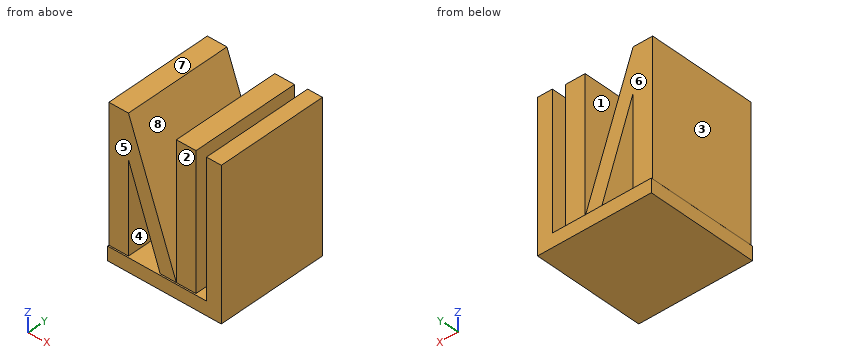
from build123d import *

# Parameters (mm, degrees)
F0_W     = 114.3
F0_H     = 152.4
F1_DEPTH = 15.24
F2_W     = 101.6
F2_H     = 14.1224
F3_DEPTH = 57.15
F4_DEPTH = 57.15
F5_W     = 20.146407
F5_H     = 137.283351
F6_DEPTH = 55.626
F7_DEPTH = 55.626


with BuildPart() as f1:
    # F0 (on Right) → F1 (new body)
    with BuildSketch(Plane.YZ):
        Rectangle(F0_W, F0_H)
    extrude(amount=F1_DEPTH)

    # F2 (on Front) → F3 (join)
    with BuildSketch(Plane.XZ):
        with Locations((-50.8, -69.1388)):
            Rectangle(F2_W, F2_H)
    extrude(amount=F3_DEPTH)

    # F2 (on Front) → F4 (join)
    with BuildSketch(Plane.XZ):
        with Locations((-50.8, -69.1388)):
            Rectangle(F2_W, F2_H)
    extrude(amount=-F4_DEPTH)

    # F5 (on Front) → F6 (join)
    with BuildSketch(Plane.XZ):
        Polygon((-101.631984, 75.205751), (-101.631984, -62.0776), (-81.485577, -62.0776), (-81.485577, 30.595854), (-81.485577, 75.205751), align=None)
        with Locations((-22.197589, 6.564075)):
            Rectangle(F5_W, F5_H)
        Polygon((-81.485577, 75.205751), (-81.485577, 30.595854), (-48.963528, -62.0776), (-32.270793, -62.0776), align=None)
    extrude(amount=F6_DEPTH)

    # F5 (on Front) → F7 (join)
    with BuildSketch(Plane.XZ):
        Polygon((-101.631984, 75.205751), (-101.631984, -62.0776), (-81.485577, -62.0776), (-81.485577, 30.595854), (-81.485577, 75.205751), align=None)
        with Locations((-22.197589, 6.564075)):
            Rectangle(F5_W, F5_H)
        Polygon((-81.485577, 75.205751), (-81.485577, 30.595854), (-48.963528, -62.0776), (-32.270793, -62.0776), align=None)
    extrude(amount=-F7_DEPTH)


solid = f1.part
Geometry: final body of the model. Coordinates: model frame, mm. Face numbers are marked on the shaded views. A direction names the side the tool comes from. Round coordinates to 2 decimals unless told otherwise and drop trailing zeros. Loops run counter-clockwise (first coordinate to the right, second up) from the corner with the lowest first, then second, coordinate; pieces in that order, holes last.
Q1. Material intervals for L1, parallel to X at y = 28.5, z = -13; L2, parallel to X at y = -22, z = 28.5; L3, parallel to X at y = 35.5, z = 60, sorted ascending.
Q2. Pull-direction query (X, two-part tool) for the marked faces 1, 2 and 3; classes: released by +X, released by -X, zero draft, split by the parting line, or undercut.
Q3. Section A-A on z = 47. Return loops of the section in (x, y), plus the area to 3 significant figures.
Q4. Pin query (flat end, axial travel): P1, Ø5, axis at x = -81.5, y = 23.5, coming from the +Z side; P2, Ø22, axis at x = -23.5, z = 5, coming from the +Y side; P3, Ø8, axis at x = -69.5, z = -16.5, coming from the +Y side; P4, Ø16, axis at x = -19, z = 31, coming from the -Y side. Return the tip coordinate at first contact, or that it passes through.
Q5. Access query for the marked faces 4, 5, 6, 7 and 8. Directions: +Z, -Z, +X, -X, +Y, -Y. A direction counts if a zero-diameter tool reaches every point of the face in a straight line with its end or side. Return the directions, or none.
Q6. Section D-D on x = -67. Return loops of the section in (y, z).
Q7. Section B-B on x = -16. Return loops of the section in (y, z), plus the area to 3 significant figures.
Evaluation:
1. L1: x = -101.63 to -81.49, -66.19 to -49.86, -32.27 to -12.12, 0 to 15.24
1. L2: x = -101.63 to -81.49, -80.75 to -64.74, -32.27 to -12.12, 0 to 15.24
1. L3: x = -101.63 to -76.03, -32.27 to -12.12, 0 to 15.24
2. face 1: undercut
2. face 2: zero draft
2. face 3: released by -X
3. outline: (-101.63, -55.63) - (-71.37, -55.63) - (-71.37, 55.63) - (-101.63, 55.63) - close; (-32.27, -55.63) - (-12.12, -55.63) - (-12.12, 55.63) - (-32.27, 55.63) - close; (0, -57.15) - (15.24, -57.15) - (15.24, 57.15) - (0, 57.15) - close
3. area: 7,350 mm2
4. P1: stops at z = 75.21
4. P2: stops at y = 55.63
4. P3: passes through
4. P4: stops at y = -55.63
5. face 4: +Y, -Y
5. face 5: +Z, -X, -Y
5. face 6: +Z, -X, +Y
5. face 7: +Z, -X, +Y, -Y
5. face 8: +Z, +Y, -Y
6. outline: (-57.15, -76.2) - (57.15, -76.2) - (57.15, -62.08) - (-57.15, -62.08) - close; (-55.63, -10.68) - (55.63, -10.68) - (55.63, 34.8) - (-55.63, 34.8) - close
7. outline: (-57.15, -76.2) - (57.15, -76.2) - (57.15, -62.08) - (55.63, -62.08) - (55.63, 75.21) - (-55.63, 75.21) - (-55.63, -62.08) - (-57.15, -62.08) - close
7. area: 16,900 mm2
